Autodesk Inventor part; units mm, degrees
ref_plane "YZ Plane" through (0, 0, 0) normal (1, 0, 0) x (0, 1, 0)
ref_plane "XZ Plane" through (0, 0, 0) normal (0, 1, 0) x (-1, 0, 0)
ref_plane "XY Plane" through (0, 0, 0) normal (0, 0, 1) x (1, 0, 0)
sketch "Sketch1" plane through (0, 0, 0) normal (1, 0, 0) x (0, 1, 0)
  circle A0 centre (0, 0) radius 4.572
  circle A1 centre (0, 0) radius 8.382
  dimension "d0" = 9.144
  dimension "d1" = 3.81
extrude "Extrusion1" add sketch "Sketch1" along normal blind 19.812
sketch "Sketch2" plane through (0, 0, 0) normal (-1, 0, 0) x (0, 0, 1)
  circle A0 centre (0, 0) radius 8.382
  circle A1 centre (0, 0) radius 7.747
  circle A2 centre (0, 0) radius 8.382
  dimension "d42" = 0
extrude "Extrusion2" add sketch "Sketch2" along normal blind 2.54 contours A0 | A1
sketch "Sketch3" plane through (-2.54, 0, 0) normal (-1, 0, 0) x (0, 0, 1)
  line L0 (19.05, 48.5955) -> (-19.05, 48.5955)
  circle A0 centre (0, 0) radius 8.382
  line L1 (8.382, 0) -> (19.05, 48.5955)
  line L2 (-8.382, 0) -> (-19.05, 48.5955)
  arc A1 (8.382, 0) -> (-8.382, 0) centre (0, 0) ccw
  line L3 (-14.3129, 44.7855) -> (14.3129, 44.7855)
  line L4 (14.3129, 44.7855) -> (6.7152, 10.176)
  arc A2 (6.7152, 10.176) -> (-6.7152, 10.176) centre (0, 0) ccw
  line L5 (-6.7152, 10.176) -> (-14.3129, 44.7855)
  dimension "d6" = 38.1
  dimension "d7" = 19.05
  dimension "d8" = 3.81
extrude "Extrusion3" add sketch "Sketch3" against normal blind 6.35 contours L1 A0 L2 L0
sketch "Sketch6" plane through (-2.54, 44.7855, -14.3129) normal (0, -1, 0) x (1, 0, 0)
  line L0 (6.35, 32.4159) -> (26.9875, 32.4159)
  line L1 (13.4874, 32.4159) -> (13.4874, 26.0989)
  line L2 (26.9875, 32.4159) -> (26.9875, -3.9117)
  point P0 (2.54, 14.3129)
  dimension "d20" = 13.5001
sketch "Sketch10" plane through (0, 0, 0) normal (1, 0, 0) x (0, 0, -1)
  circle A0 centre (0, 0) radius 1.4542
  line L0 (-4.572, 1.4542) -> (4.572, 1.4542)
  line L1 (4.572, 1.4542) -> (4.572, -1.4542)
  line L2 (4.572, -1.4542) -> (-4.572, -1.4542)
  line L3 (-4.572, -1.4542) -> (-4.572, 1.4542)
  circle A1 centre (0, 0) radius 4.572
  dimension "d43" = 0
  dimension "d44" = 0
extrude "Extrusion7" cut sketch "Sketch10" against normal blind 22.225 contours A0 | A0 L0 A1 L2 | A0 L2 A1 L0 | A1 L3 L0 | L0 L1 A1 | A1 L1 L2 | L2 L3 A1
sketch "Sketch13" plane through (-2.54, 48.5955, 19.05) normal (0, 1, 0) x (1, 0, 0)
  line L0 (4.6355, 36.83) -> (1.7145, 36.83)
  line L1 (1.7145, 36.83) -> (1.7145, 33.909)
  line L2 (1.7145, 33.909) -> (4.6355, 33.909)
  line L3 (4.6355, 33.909) -> (4.6355, 36.83)
  line L4 (6.35, 38.1) -> (6.35, 0)
  line L5 (0, 38.1) -> (6.35, 38.1)
  line L6 (4.6228, 4.191) -> (1.7018, 4.191)
  line L7 (1.7018, 4.191) -> (1.7018, 1.27)
  line L8 (1.7018, 1.27) -> (4.6228, 1.27)
  line L9 (4.6228, 1.27) -> (4.6228, 4.191)
  line L10 (0, 0) -> (6.35, 0)
  line L11 (0, 0) -> (0, 38.1)
  line L12 (0, 0) -> (6.35, 0)
  line L13 (6.35, 38.1) -> (6.35, 0)
  line L14 (0, 38.1) -> (6.35, 38.1)
  point P0 (2.54, 19.05)
  dimension "d32" = 2.921
  dimension "d33" = 2.921
  dimension "d34" = 1.7145
  dimension "d35" = 1.27
  dimension "d36" = 2.921
  dimension "d37" = 2.921
  dimension "d38" = 1.7272
  dimension "d39" = 1.27
extrude "Extrusion9" add sketch "Sketch13" along normal blind 3.81 contours L3 L2 L1 L0 | L4 L10 L11 L5 | L9 L8 L7 L6
sketch "Sketch14" plane through (0, 0, 0) normal (-1, 0, 0) x (0, 0, 1)
  arc A0 (4.3346, -1.4542) -> (4.572, 0) centre (0, 0) ccw
  line L0 (4.3346, -1.4542) -> (4.572, -1.4542)
  line L1 (4.572, -1.4542) -> (4.572, 0)
  arc A1 (4.572, 0) -> (4.3346, 1.4542) centre (0, 0) ccw
  line L2 (4.572, 0) -> (4.572, 1.4542)
  line L3 (4.572, 1.4542) -> (4.3346, 1.4542)
  arc A2 (-4.572, 0) -> (-4.3346, -1.4542) centre (0, 0) ccw
  line L4 (-4.572, 0) -> (-4.572, -1.4542)
  line L5 (-4.572, -1.4542) -> (-4.3346, -1.4542)
  arc A3 (-4.3346, 1.4542) -> (-4.572, 0) centre (0, 0) ccw
  line L6 (-4.3346, 1.4542) -> (-4.572, 1.4542)
  line L7 (-4.572, 1.4542) -> (-4.572, 0)
extrude "Extrusion10" add sketch "Sketch14" along normal blind 2.54
sketch "Sketch15" plane through (-2.54, 0, 0) normal (-1, 0, 0) x (0, 0, 1)
  circle A0 centre (0, 0) radius 41.275
  circle A1 centre (0, 0) radius 44.45
  dimension "d47" = 82.55
  dimension "d48" = 88.9
extrude "Extrusion11" add sketch "Sketch15" against normal blind 2.54
sketch "Sketch16" plane through (0, 0, 0) normal (1, 0, 0) x (0, 0, -1)
  circle A0 centre (0, 0) radius 44.45
  circle A1 centre (0, 0) radius 41.275
  dimension "d51" = 82.55
extrude "Extrusion12" add sketch "Sketch16" along normal blind 25.4
sketch "Sketch19" plane through (-2.54, 0, 0) normal (-1, 0, 0) x (0, 0, 1)
  line L0 (4.3346, 1.4542) -> (-4.3346, 1.4542)
  arc A0 (-16.671, 37.7585) -> (16.671, 37.7585) centre (0, 0) ccw
  line L1 (-4.3346, 1.4542) -> (-41.2494, 1.4542)
  line L2 (4.3346, 1.4542) -> (41.2494, 1.4542)
  circle A1 centre (0, 0) radius 8.382
  line L3 (-4.3346, -1.4542) -> (4.3346, -1.4542)
  line L4 (4.3346, 1.4542) -> (-4.3346, 1.4542)
  line L5 (-41.2494, -1.4542) -> (41.2494, -1.4542)
extrude "Extrusion14" add sketch "Sketch19" against normal blind 6.35 contours L2 A1 L5 L3 L1 L0 | L2 A0 L5 A1 | A1 L5 A0 L1
sketch "Sketch20" plane through (3.81, 0, 0) normal (1, 0, 0) x (0, 0, -1)
  arc A0 (4.3346, -1.4542) -> (4.3346, 1.4542) centre (0, 0) ccw
  line L0 (4.3346, 1.4542) -> (-4.3346, 1.4542)
  arc A1 (-4.3346, 1.4542) -> (-4.3346, -1.4542) centre (0, 0) ccw
  line L1 (-4.3346, -1.4542) -> (4.3346, -1.4542)
extrude "Extrusion15" cut sketch "Sketch20" against normal blind 6.35
sketch "Sketch21" plane through (-2.54, 0, 0) normal (-1, 0, 0) x (0, 0, 1)
  arc A0 (-8.2549, -1.4542) -> (8.2549, -1.4542) centre (0, 0) ccw
  line L0 (1.8492, -8.1755) -> (1.8492, -41.2336)
  arc A1 (-41.2494, -1.4542) -> (41.2494, -1.4542) centre (0, 0) ccw
  line L1 (-1.8492, -41.2336) -> (-1.8492, -8.1755)
  arc A2 (-1.8492, -8.1755) -> (1.8492, -8.1755) centre (0, 0) ccw
  arc A3 (-1.8492, -41.2336) -> (1.8492, -41.2336) centre (0, 0) ccw
extrude "Extrusion16" add sketch "Sketch21" against normal blind 6.35
sketch "Sketch22" plane through (-2.54, 48.5955, 19.05) normal (0, 1, 0) x (1, 0, 0)
  point P0 (2.54, 19.05)
sketch "Sketch23" plane through (3.81, 0, 0) normal (1, 0, 0) x (0, 0, -1)
  line L0 (19.05, 52.4055) -> (-19.05, 52.4055)
  line L1 (-19.05, 48.5955) -> (-19.05, 52.4055)
  line L2 (19.05, 52.4055) -> (-19.05, 52.4055)
  line L3 (-19.05, 52.4055) -> (-19.05, 48.5955)
  line L4 (-19.05, 48.5955) -> (19.05, 48.5955)
  line L5 (19.05, 48.5955) -> (19.05, 52.4055)
  point P0 (0, 0)
extrude "Extrusion17" add sketch "Sketch23" along normal blind 19.05
properties part number "BasicThrustMotorHousing"
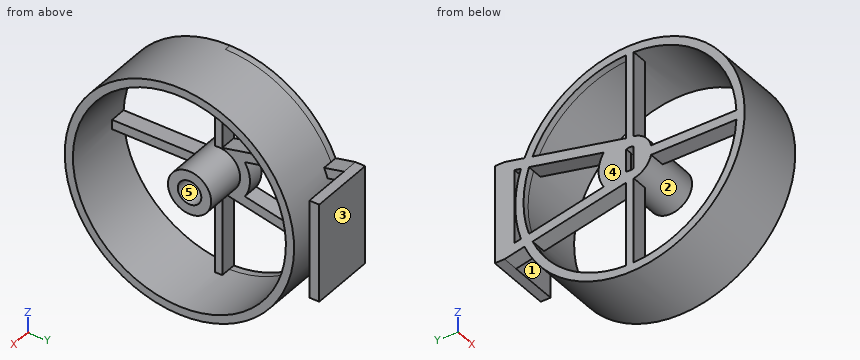
The model under review builds one solid part; all positions refer to its coordinate system, in mm. Face numbers are marked on the shaded views. A direction names the side the tool comes from. Give positions to 0.01 mm unless a question says otherwise; leave off trailing zeros. Write each loop counter-clockwise with the first axis right and the second up, starting at its lowest first coordinate (ties: lowest second). Pieces come first, ordered by that corner, then holes. Notation, with made-up numbers: M 54.25,83.25 L 72.25,83.25 A32 ccw 72.25,121.25 Z; hole C 86,-22 d5. An arc over 180 degrees is marked long. Answer in a Markdown table with one row per item.
Item 1: Tool access review of the marked faces 1, 2 and 3: name each direction out of +Z, -Z, +X, -X, +Y, -Y from which nothing blocks a thin tool from reaching the whole face with its end or side.
Check sheet entries:
| item | result |
|---|---|
| face 1 | +Z, -Z, +X |
| face 2 | +X |
| face 3 | +Z, -Z, +X, -X, +Y |
Item 2: For P1, Ø1.8, axis at y = -32.5, z = 0.5, coming from the +X side; P2, Ø3, axis at x = 2, z = 23, coming from the -Y side; P3, Ø3, axis at x = 2, y = -18, coming from the +Z side, all flat-tipped, find the tip position at first contact; note any pin that passes through.
Check sheet entries:
| item | result |
|---|---|
| P1 | x = 3.81 |
| P2 | y = -38.9 |
| P3 | z = 41.27 |
Item 3: Add section C-C on x = 7.25. State how many separate pieces and enclosed holes the cut face has, plus the area to 3 significant figures.
Check sheet entries:
| item | result |
|---|---|
| separate pieces | 3 |
| enclosed holes | 2 |
| area | 1,160 mm2 |
Item 4: Add section B-B on z = -29. Give the boundary of the cut face in (x, y).
Check sheet entries:
| item | result |
|---|---|
| outline | M -2.54,-33.69 L 25.4,-33.69 L 25.4,-29.37 L -2.54,-29.37 Z; M -2.54,-1.45 L 3.81,-1.45 L 3.81,1.45 L -2.54,1.45 Z; M -2.54,29.37 L 25.4,29.37 L 25.4,33.69 L -2.54,33.69 Z |
Item 5: For line 1 along Z through (x, y) = (9.5, 0) (3 decimals); line 2 along Z through (x, y) = (8.75, -0.5); line 3 along Y through (x, z) = (4.5, -4), list the stretches that pass through material, from the lowest coordinate up.
Check sheet entries:
| item | result |
|---|---|
| line 1 | -44.45 to -41.275, -8.382 to -4.572, 4.572 to 8.382, 41.275 to 44.45 |
| line 2 | -44.45 to -41.27, -8.37 to -4.54, 4.54 to 8.37, 41.27 to 44.45 |
| line 3 | -44.27 to -41.08, -7.37 to -2.21, 2.21 to 7.37, 41.08 to 44.27, 48.6 to 52.41 |
Item 6: Draft analysis for pull direction Z (two halves, no side actions). For the marked faces 4 and 5, state which applies: +Z half, -Z half, draft (parallel to the pull), parting line (faces both ways), or undercut.
Check sheet entries:
| item | result |
|---|---|
| face 4 | draft |
| face 5 | undercut |
